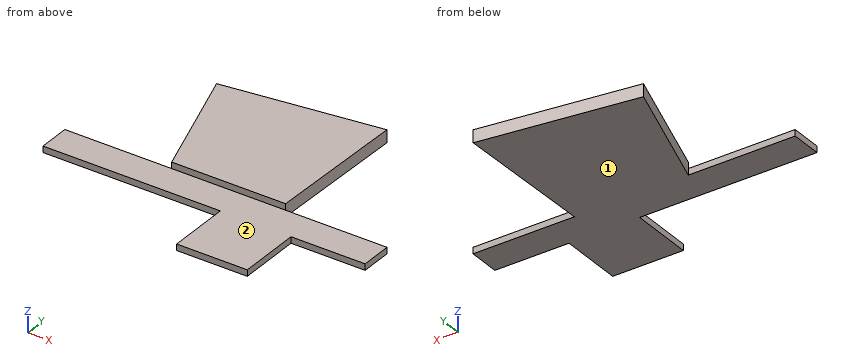
from build123d import *

# Parameters (mm, degrees)
F1_DEPTH = 1
F2_W     = 5.6130217854
F2_H     = 2.4976935238
F2_W_2   = 14.08868609
F2_W_3   = 5.8936730493
F2_H_2   = 4.9955896102
F3_DEPTH = 0.5


with BuildPart() as f1:
    # F0 (on Top) → F1 (new body)
    with BuildSketch(Plane.XY):
        Polygon((-12.1924033149, 9.6513108647), (-9.05, 0), (-5.4919267763, 4.3473211306), align=None)
        Polygon((-5.4919267763, 4.3473211306), (0, 0), (0.1970994475, 11.2982809227), align=None)
        Polygon((-12.1924033149, 9.6513108647), (-5.4919267763, 4.3473211306), (0.1970994475, 11.2982809227), align=None)
        Polygon((-9.05, 0), (0, 0), (-5.4919267763, 4.3473211306), align=None)
    extrude(amount=F1_DEPTH)

    # F2 (on Top) → F3 (join)
    with BuildSketch(Plane.XY):
        with Locations((-0.6455987459, -1.2488467619)):
            Rectangle(F2_W, F2_H)
        with Locations((-10.4964526836, -1.2488467619)):
            Rectangle(F2_W_2, F2_H)
        with Locations((5.1077486714, -1.2488467619)):
            Rectangle(F2_W_3, F2_H)
        with Locations((-0.6455987459, -4.9954883289)):
            Rectangle(F2_W, F2_H_2)
    extrude(amount=F3_DEPTH)


solid = f1.part
Could you check a few things on this model? Use its own coordinates, in mm. Face numbers are marked on the shaded views. A direction names the side the tool comes from. Give positions to 0.01 mm unless a question says otherwise; leave off trailing zeros. Order: outer loops, then holes, each group sorted by start corner. A loop starts at its lowest first (then second) coordinate and runs counter-clockwise, first axis right, second up.
Item 1: If we section it at A-A, the plane x = -10.5: Write out the boundary of the cut face in (y, z).
Item 2: If we section it at B-B, the plane z = 0.3: Write out the boundary of the cut face in (x, y).
Item 3: If we section it at C-C, the plane x = -5.25: Write out the boundary of the cut face in (y, z).
Item 4: For the marked faces 1 and 2, which set-ups out of +Z, -Z, +X, -X, +Y, -Y let a thin tool reach every point of the face, with its end or its side?
Item 5: If we section it at D-D, the plane y = 5.5: Write out the boundary of the cut face in (x, z), plus the area to 3 significant figures.
Item 6: I'm going to push flat-ended pins straight in: pin 1 (10 mm diameter, centred on x = 2, y = -2.5, fed in from -Z); pin 2 (6 mm diameter, centred on x = -0.5, y = -3.5, fed in from +Z). Where does each tip first touch, or does it pass through?
Item 7: I need wall thicknesses on line 1 (X direction, y = -6.5, z = 0.2); line 2 (Z direction, x = -6.75, y = -1.5); line 3 (X direction, y = 2.5, z = 0.6). Which ranges of each line are inside material? Lowest first, please.
Values:
1. outline: (-2.5, 0) - (0, 0) - (0, 0.5) - (-2.5, 0.5) - close; (4.45, 0) - (9.88, 0) - (9.88, 1) - (4.45, 1) - close
2. outline: (-17.54, -2.5) - (-3.45, -2.5) - (-3.45, -7.49) - (2.16, -7.49) - (2.16, -2.5) - (8.05, -2.5) - (8.05, 0) - (0, 0) - (0.2, 11.3) - (-12.19, 9.65) - (-9.05, 0) - (-17.54, 0) - close
3. outline: (-2.5, 0) - (10.57, 0) - (10.57, 1) - (0, 1) - (0, 0.5) - (-2.5, 0.5) - close
4. face 1: -Z, +X, -X, +Y, -Y
4. face 2: +Z, +X, -X, -Y
5. outline: (-10.84, 0) - (0.1, 0) - (0.1, 1) - (-10.84, 1) - close
5. area: 10.9 mm2
6. pin 1: stops at z = 0
6. pin 2: stops at z = 0.5
7. line 1: x = -3.45 to 2.16
7. line 2: z = 0 to 0.5
7. line 3: x = -9.86 to 0.04
